Read the model definition and answer for the solid it produces. Units are mm, in the model's axes. Face numbers are marked on the shaded views. A direction names the side the tool comes from. Coordinates: 2 decimals unless noted, no trailing zeros. Loops run counter-clockwise (first coordinate to the right, second up) from the corner with the lowest first, then second, coordinate; pieces in that order, holes last. Notation, with made-up numbers: M 9,-6 L 66,-6 A29 ccw 66,17 Z; hole C 81,20 d11. An arc over 180 degrees is marked long. One line per item, written item: value. Start each with the question number.
1. Consider probe 1 along X at (y, z) = (27.1, 27); probe 2 along Z at (x, y) = (-51, 7); probe 3 along X at (y, z) = (11, 7). Determine where each line is inside the solid, lowest interval first.
2. The part is cut by section B-B (x = -43). Write down the section's boundary in (y, z), then the cut area to 3 significant figures.
3. Determine the mould class of the marked faces 3 and 4 for opening direction Z: +Z half, -Z half, draft (parallel to the pull), parting line (faces both ways), or undercut.
4. For the marked faces 1 and 2, determine the directions among +Z, -Z, +X, -X, +Y, -Y from which every point of the face is accessible in a straight line to the end or side of a thin tool.
5. The part is cut by section A-A (y = 15.5). Write down the section's boundary in (x, z).
6. Flat-ended cylindrical pins translate along their axes: pin 1 (1.5 mm diameter, centred on x = -61, z = -1.5, fed in from +Y); pin 2 (5 mm diameter, centred on x = -59, z = 27, fed in from -Y); pin 3 (1 mm diameter, centred on y = 17.5, z = -17.5, fed in from -X). Find the tip coordinate at first contact, or state that the pin passes through.
```python
from build123d import *

# Parameters (mm, degrees)
SKETCH1_W      = 126
SKETCH1_H      = 46
EXTRUDE1_DEPTH = 3
SKETCH2_W      = 126
SKETCH2_H      = 46
SKETCH2_W_2    = 120
SKETCH2_H_2    = 40
EXTRUDE2_DEPTH = 25
SKETCH3_R      = 1.5
EXTRUDE3_DEPTH = 3
SKETCH4_W      = 40
SKETCH4_H      = 15
EXTRUDE4_DEPTH = 3


with BuildPart() as part:
    # Sketch1 → Extrude1 (new body)
    with BuildSketch(Plane(origin=(0, 0, 0), x_dir=(1, 0, 0), z_dir=(0, 1, 0))):
        Rectangle(SKETCH1_W, SKETCH1_H)
    extrude(amount=EXTRUDE1_DEPTH)

    # Sketch2 → Extrude2 (add)
    with BuildSketch(Plane(origin=(0, 3, 0), x_dir=(1, 0, 0), z_dir=(0, 1, 0))):
        Rectangle(SKETCH2_W, SKETCH2_H)
        Rectangle(SKETCH2_W_2, SKETCH2_H_2, mode=Mode.SUBTRACT)
    extrude(amount=EXTRUDE2_DEPTH)

    # Sketch3 → Extrude3 (add)
    # profile 1 of 4: a face of its own
    with BuildSketch(Plane(origin=(0, 28, 0), x_dir=(1, 0, 0), z_dir=(0, 1, 0))):
        with BuildLine():
            Line((63, -23), (63, -27))
            ThreePointArc((63, -27), (61.828427125, -29.828427125), (59, -31))
            ThreePointArc((59, -31), (56.171572875, -29.828427125), (55, -27))
            Line((55, -27), (55, -23))
            Line((55, -23), (63, -23))
        make_face()
        with Locations(Location((59, -27, 0), (0, 0, 270))):
            Circle(SKETCH3_R, mode=Mode.SUBTRACT)
    # profile 2 of 4: a face of its own
    with BuildSketch(Plane(origin=(0, 28, 0), x_dir=(1, 0, 0), z_dir=(0, 1, 0))):
        with BuildLine():
            Line((-63, -23), (-55, -23))
            Line((-55, -23), (-55, -27))
            ThreePointArc((-55, -27), (-56.171572875, -29.828427125), (-59, -31))
            ThreePointArc((-59, -31), (-61.828427125, -29.828427125), (-63, -27))
            Line((-63, -27), (-63, -23))
        make_face()
        with Locations(Location((-59, -27, 0), (0, 0, 270))):
            Circle(SKETCH3_R, mode=Mode.SUBTRACT)
    # profile 3 of 4: a face of its own
    with BuildSketch(Plane(origin=(0, 28, 0), x_dir=(1, 0, 0), z_dir=(0, 1, 0))):
        with BuildLine():
            Line((55, 27), (55, 23))
            Line((55, 23), (63, 23))
            Line((63, 23), (63, 27))
            ThreePointArc((63, 27), (61.828427125, 29.828427125), (59, 31))
            ThreePointArc((59, 31), (56.171572875, 29.828427125), (55, 27))
        make_face()
        with Locations(Location((59, 27, 0), (0, 0, 90))):
            Circle(SKETCH3_R, mode=Mode.SUBTRACT)
    # profile 4 of 4: a face of its own
    with BuildSketch(Plane(origin=(0, 28, 0), x_dir=(1, 0, 0), z_dir=(0, 1, 0))):
        with BuildLine():
            Line((-55, 27), (-55, 23))
            Line((-55, 23), (-63, 23))
            Line((-63, 23), (-63, 27))
            ThreePointArc((-63, 27), (-61.828427125, 29.828427125), (-59, 31))
            ThreePointArc((-59, 31), (-56.171572875, 29.828427125), (-55, 27))
        make_face()
        with Locations(Location((-59, 27, 0), (0, 0, 90))):
            Circle(SKETCH3_R, mode=Mode.SUBTRACT)
    extrude(amount=-EXTRUDE3_DEPTH)

    # Sketch4 → Extrude4 (cut)
    with BuildSketch(Plane(origin=(-60, 0, 0), x_dir=(0, 0, -1), z_dir=(1, 0, 0))):
        with Locations((0, 20.5)):
            Rectangle(SKETCH4_W, SKETCH4_H)
    extrude(amount=-EXTRUDE4_DEPTH, mode=Mode.SUBTRACT)


solid = part.part
```
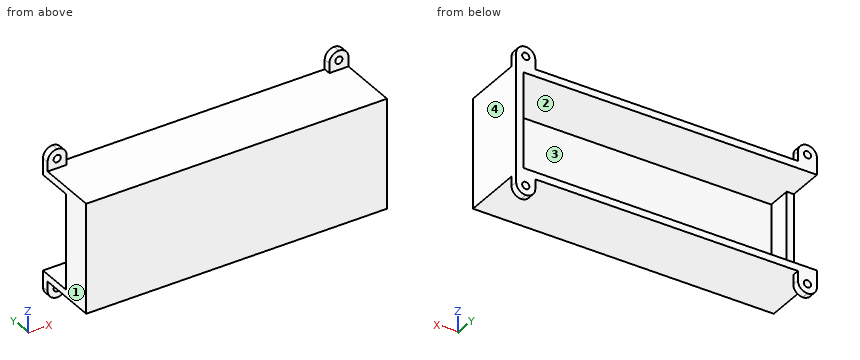
Answer block:
1. probe 1: x = -63 to -60.5, -57.5 to -55, 55 to 57.5, 60.5 to 63
1. probe 2: z = -23 to -20, 20 to 23
1. probe 3: x = -63 to -60, 60 to 63
2. outline: M 0,-23 L 28,-23 L 28,-20 L 3,-20 L 3,20 L 28,20 L 28,23 L 0,23 Z
2. area: 288 mm2
3. face 3: undercut
3. face 4: draft
4. face 1: +Z, -Z, -X, +Y, -Y
4. face 2: +Y
5. outline: M -63,-23 L 63,-23 L 63,23 L -63,23 L -63,20 L 60,20 L 60,-20 L -63,-20 Z
6. pin 1: stops at y = 13
6. pin 2: stops at y = 25
6. pin 3: stops at x = 60
